from build123d import *

# Parameters (mm, degrees)
SKETCH1_R           = 7.5
SKETCH1_R_2         = 2
BOSS_EXTRUDE1_DEPTH = 2
FILLET1_R           = 0.5
CHAMFER1_SIZE       = 2


with BuildPart() as part:
    # Sketch1 → Boss-Extrude1 (new, symmetric)
    with BuildSketch(Plane(origin=(0, 0, 0), x_dir=(1, 0, 0), z_dir=(0, 1, 0))):
        with Locations(Location((0, 0, 0), (0, 0, 270))):
            Circle(SKETCH1_R)
        with Locations(Location((0, 0, 0), (0, 0, 270))):
            Circle(SKETCH1_R_2, mode=Mode.SUBTRACT)
    extrude(amount=BOSS_EXTRUDE1_DEPTH, both=True)

    # Fillet1
    fillet1_edges = [part.edges().sort_by_distance(p)[0] for p in [
        (0, -2, -7.5),
        (0, 2, -7.5),
    ]]
    fillet(fillet1_edges, radius=FILLET1_R)

    # Chamfer1
    chamfer1_edges = [part.edges().sort_by_distance(p)[0] for p in [
        (0, 2, -2),
    ]]
    chamfer(chamfer1_edges, length=CHAMFER1_SIZE)


solid = part.part
CAD build for the part. Positions are in the model's coordinates, mm. Coordinates: 2 decimals unless noted, no trailing zeros. Order: outer loops, then holes, each group sorted by start corner. A loop starts at its lowest first (then second) coordinate and runs counter-clockwise, first axis right, second up.
Item 1: Two-plate mould, pull along X, no slides. Class faces 1 (the face through (0.33, 0.021, -7.493)), 2 (the face through (-2, -1, 0)), 3 (the face through (-3, 2, 3)): +X half, -X half, draft (parallel to the pull), parting line (faces both ways), or undercut.
Check sheet entries:
face 1: parting line
face 2: undercut
face 3: draft
Item 2: Band-saw the part on C-C on y = -0.85. List the corners of the cut face in (x, z).
Check sheet entries:
outline: circle Ø15 at (0, 0); hole circle Ø4 at (0, 0)
Item 3: Band-saw the part on B-B on x = 0. List the corners of the cut face in (y, z).
Check sheet entries:
outline: (-2, -7) arc R0.5 ccw to (-1.5, -7.5) - (1.5, -7.5) arc R0.5 ccw to (2, -7) - (2, -4) - (0, -2) - (-2, -2) - close; (-2, 2) - (0, 2) - (2, 4) - (2, 7) arc R0.5 ccw to (1.5, 7.5) - (-1.5, 7.5) arc R0.5 ccw to (-2, 7) - close
Item 4: Drill centre lines: L1, parallel to X at y = -1.2, z = 0; L2, parallel to X at y = -1.1, z = -0.75; L3, parallel to Z at x = -0.5, y = -1.55. Where is each one in solid material? Low to high.
Check sheet entries:
L1: x = -7.5 to -2, 2 to 7.5
L2: x = -7.46 to -1.85, 1.85 to 7.46
L3: z = -7.48 to -1.94, 1.94 to 7.48
Item 5: Band-saw the part on D-D on y = 0.6. List the corners of the cut face in (x, z), plus the area to 3 significant figures.
Check sheet entries:
outline: circle Ø15 at (0, 0); hole circle Ø5.2 at (0, 0)
area: 155 mm2
Item 6: Pin check, flat tips, straight feed: pin 1 Ø6.5 at (x, z) = (0, 0) entering from +Y; pin 2 Ø2 at (x, z) = (-1, -1) entering from +Y; pin 3 Ø1.5 at (y, z) = (-1, -3.5) entering from +X; pin 4 Ø8 at (x, z) = (5, 5.5) entering from +Y. Stop position of each tip, or through.
Check sheet entries:
pin 1: stops at y = 1.25
pin 2: stops at y = 0.41
pin 3: stops at x = 6.98
pin 4: stops at y = 2
Item 7: Band-saw the part on A-A on z = 0. List the corners of the cut face in (x, y), plus the area to 3 significant figures.
Check sheet entries:
outline: (-7.5, -1.5) arc R0.5 ccw to (-7, -2) - (-2, -2) - (-2, 0) - (-4, 2) - (-7, 2) arc R0.5 ccw to (-7.5, 1.5) - close; (2, -2) - (7, -2) arc R0.5 ccw to (7.5, -1.5) - (7.5, 1.5) arc R0.5 ccw to (7, 2) - (4, 2) - (2, 0) - close
area: 39.8 mm2
